Input: part model. Units: mm. Frame: model coordinates. Face numbers are marked on the shaded views. A direction names the side the tool comes from. Round coordinates to 2 decimals unless told otherwise and drop trailing zeros. Order: outer loops, then holes, each group sorted by start corner. A loop starts at its lowest first (then second) coordinate and runs counter-clockwise, first axis right, second up. Notation, with made-up numbers: (54, 78.25) -> (63, 78.25) arc R23 cw to (63, 86.25) -> close; hole circle Ø10 at (32, 68.5). An arc over 180 degrees is marked (long way). Use a Markdown table: item, result.
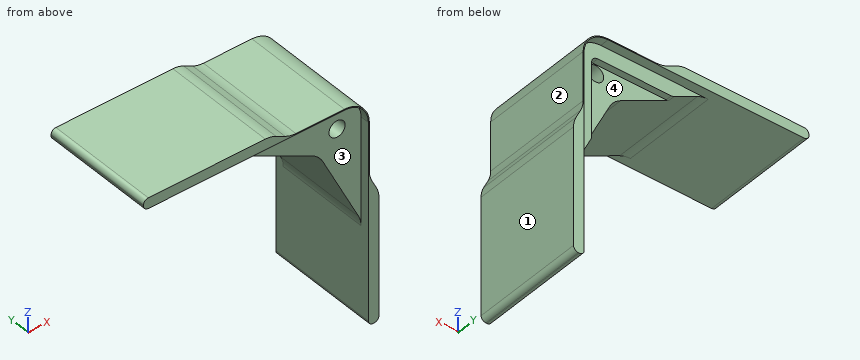
from build123d import *
from build123d.topology import SkipClean

# Parameters (mm, degrees)
SKETCH1_R           = 4.28625
BOSS_EXTRUDE1_DEPTH = 50.8
FILLET2_R           = 2.54
SKETCH7_W           = 42.968170869
SKETCH7_H           = 42.968170869
CUT_EXTRUDE3_DEPTH  = 3.429
FILLET9_R           = 3.175
BOSS_EXTRUDE2_DEPTH = 30.1625
CUT_EXTRUDE4_DEPTH  = 163.081683034
FILLET10_R          = 12.7


with BuildPart() as part:
    # Sketch1 → Boss-Extrude1 (new body)
    with BuildSketch(Plane(origin=(0, 0, 0), x_dir=(1, 0, 0), z_dir=(0, 1, 0))):
        with BuildLine():
            Line((12.7, 53.934971632), (-9.469611004, 9.469611004))
            Line((-9.469611004, 9.469611004), (-53.934971632, -12.7))
            Line((-53.934971632, -12.7), (-106.3752, -12.7))
            Line((-106.3752, -12.7), (-106.3752, -18.288))
            Line((-106.3752, -18.288), (0, -18.288))
            ThreePointArc((0, -18.288), (12.931568814, -12.931568814), (18.288, 0))
            Line((18.288, 0), (18.288, 106.3752))
            Line((18.288, 106.3752), (12.7, 106.3752))
            Line((12.7, 106.3752), (12.7, 53.934971632))
        make_face()
        with Locations(Location((0, 0, 0), (0, 0, 270))):
            Circle(SKETCH1_R, mode=Mode.SUBTRACT)
    extrude(amount=BOSS_EXTRUDE1_DEPTH)

    # Fillet2
    fillet2_edges = [part.edges().sort_by_distance(p)[0] for p in [
        (12.7, 25.4, -106.3752),
        (18.288, 25.4, -106.3752),
        (-106.3752, 25.4, 18.288),
        (-106.3752, 25.4, 12.7),
    ]]
    fillet(fillet2_edges, radius=FILLET2_R)

    # Sketch7 → Cut-Extrude3 (cut)
    with BuildSketch(Plane(origin=(0, 50.8, 0), x_dir=(1, 0, 0), z_dir=(0, 1, 0))):
        with Locations((-16.658085435, 16.658085435)):
            Rectangle(SKETCH7_W, SKETCH7_H)
    extrude(amount=-CUT_EXTRUDE3_DEPTH, mode=Mode.SUBTRACT)

    # Fillet9
    fillet9_edges = [part.edges().sort_by_distance(p)[0] for p in [
        (4.826, 49.0855, -38.142170869),
        (4.826, 49.0855, 4.826),
        (-38.142170869, 49.0855, 4.826),
    ]]
    fillet(fillet9_edges, radius=FILLET9_R)

    # Sketch8 → Boss-Extrude2 (add, symmetric)
    with SkipClean():  # the faces are left unmerged after this step: merging them gives an invalid solid
        with BuildSketch(Plane(origin=(0, 25.4, 0), x_dir=(1, 0, 0), z_dir=(0, 1, 0))):
            with BuildLine():
                Line((0, -12.7), (-103.8352, -12.7))
                ThreePointArc((-103.8352, -12.7), (-105.631251224, -13.443948776), (-106.3752, -15.24))
                Line((-106.3752, -15.24), (-106.3752, -15.748))
                ThreePointArc((-106.3752, -15.748), (-105.631251224, -17.544051224), (-103.8352, -18.288))
                Line((-103.8352, -18.288), (0, -18.288))
                ThreePointArc((0, -18.288), (12.931568814, -12.931568814), (18.288, 0))
                Line((18.288, 0), (18.288, 103.8352))
                ThreePointArc((18.288, 103.8352), (17.544051224, 105.631251224), (15.748, 106.3752))
                Line((15.748, 106.3752), (15.24, 106.3752))
                ThreePointArc((15.24, 106.3752), (13.443948776, 105.631251224), (12.7, 103.8352))
                Line((12.7, 103.8352), (12.7, 0))
                ThreePointArc((12.7, 0), (8.980256121, -8.980256121), (0, -12.7))
            make_face()
        extrude(amount=BOSS_EXTRUDE2_DEPTH, both=True)
    add(part.part.scale(1), mode=Mode.REPLACE)  # the faces are merged on a copy

    # Sketch9 → Cut-Extrude4 (cut, through all)
    with BuildSketch(Plane(origin=(0, 55.5625, 0), x_dir=(1, 0, 0), z_dir=(0, 1, 0))):
        with BuildLine():
            Line((-28.673096282, -13.208), (-38.862, -18.288))
            Line((-38.862, -18.288), (0, -18.288))
            ThreePointArc((0, -18.288), (12.931568814, -12.931568814), (18.288, 0))
            Line((18.288, 0), (18.288, 38.862))
            Line((18.288, 38.862), (13.208, 28.673096282))
            Line((13.208, 28.673096282), (13.208, 0))
            ThreePointArc((13.208, 0), (9.339466366, -9.339466366), (0, -13.208))
            Line((0, -13.208), (-28.673096282, -13.208))
        make_face()
    extrude(amount=-CUT_EXTRUDE4_DEPTH, mode=Mode.SUBTRACT)

    # Fillet10
    fillet10_edges = [part.edges().sort_by_distance(p)[0] for p in [
        (13.208, 25.4, -28.673096282),
        (18.288, 25.4, -38.862),
        (-38.862, 25.4, 18.288),
        (-28.673096282, 25.4, 13.208),
        (12.7, 25.4, -53.934971632),
        (-53.934971632, 25.4, 12.7),
        (-9.469611004, 23.6855, -9.469611004),
    ]]
    fillet(fillet10_edges, radius=FILLET10_R)


solid = part.part
1) Cut plane B-B on z = -11. Return loops of the section in (x, y), and give its area (3 significant figures).
Answer key:
| item | result |
|---|---|
| outline | (-9.03, 0) -> (12.7, 0) -> (12.7, -4.76) -> (13.21, -4.76) -> (13.21, 55.56) -> (12.7, 55.56) -> (12.7, 50.8) -> (4.83, 50.8) -> (4.83, 47.37) -> (-9.03, 47.37) -> close |
| area | 1,090 mm^2 |
2) Cut plane A-A on y = 14. Return loops of the section in (x, z), and give its area (3 significant figures).
Answer key:
| item | result |
|---|---|
| outline | (-106.38, 15.24) arc R2.54 ccw to (-103.84, 12.7) -> (-56.93, 12.7) arc R12.7 cw to (-51.26, 11.37) -> (-13.27, -7.57) arc R12.7 cw to (-7.57, -13.27) -> (11.37, -51.26) arc R12.7 cw to (12.7, -56.93) -> (12.7, -103.84) arc R2.54 ccw to (15.24, -106.38) -> (15.75, -106.38) arc R2.54 ccw to (18.29, -103.84) -> (18.29, -41.85) arc R12.7 ccw to (16.95, -36.19) -> (14.54, -31.35) arc R12.7 cw to (13.21, -25.68) -> (13.21, 0) arc R13.21 ccw to (0, 13.21) -> (-25.68, 13.21) arc R12.7 cw to (-31.35, 14.54) -> (-36.19, 16.95) arc R12.7 ccw to (-41.85, 18.29) -> (-103.84, 18.29) arc R2.54 ccw to (-106.38, 15.75) -> close; hole circle Ø8.57 at (0, 0) |
| area | 2,240 mm^2 |
3) Cut plane C-C on x = -43.5. Return loops of the section in (y, z).
Answer key:
| item | result |
|---|---|
| outline | (-4.76, 12.7) -> (0, 12.7) -> (0, 7.5) -> (50.8, 7.5) -> (50.8, 12.7) -> (55.56, 12.7) -> (55.56, 18.29) -> (-4.76, 18.29) -> close |
4) Cut plane D-D on x = -22. Return loops of the section in (y, z), and give its area (3 significant figures).
Answer key:
| item | result |
|---|---|
| outline | (-4.76, 12.7) -> (0, 12.7) -> (0, -3.22) -> (47.37, -3.22) -> (47.37, 4.83) -> (50.8, 4.83) -> (50.8, 12.7) -> (55.56, 12.7) -> (55.56, 13.21) -> (-4.76, 13.21) -> close |
| area | 812 mm^2 |
5) Ray query, probe 1 along X at (y, z) = (16, -58.5); probe 2 along X at (y, z) = (33.5, 0). Return the intervals inside material, ascending.
Answer key:
| item | result |
|---|---|
| probe 1 | x = 12.7 to 18.29 |
| probe 2 | x = -28.46 to -4.29, 4.29 to 13.21 |
6) Set-up query: the marked faces 1, 2, 3 and 4. Return all of +Z, -Z, +X, -X, +Y, -Y with unobstructed straight access to the full face (end or side cutting, diameter ignored); none if empty.
Answer key:
| item | result |
|---|---|
| face 1 | +Z, -Z, +X, +Y, -Y |
| face 2 | +Z, +X, +Y, -Y |
| face 3 | -Z, -X, -Y |
| face 4 | -Z, -X, +Y |
7) Contact query for flat-ended pins moving along their axis: P1, Ø2.5, axis at x = -24.5, y = 49, coming from the -Z side; P2, Ø20.5, axis at x = -18, y = 37.5, coming from the +Z side; P3, Ø20.5, axis at y = 22.5, z = -8, coming from the +X side; P4, Ø13, axis at x = -16.5, z = -20, coming from the +Y side. Output: stop coordinate, or through.
Answer key:
| item | result |
|---|---|
| P1 | stops at z = 4.83 |
| P2 | stops at z = 13.47 |
| P3 | stops at x = 13.21 |
| P4 | passes through |
